Can you work these out from the model? Positions are in its coordinate system, mm. Face numbers are marked on the shaded views. Give positions to 0.01 mm unless a question says otherwise; leave off trailing zeros. Write each loop counter-clockwise with the first axis right and the second up, starting at its lowest first coordinate (ties: lowest second). Pieces come first, ordered by that corner, then holes. Notation, with made-up numbers: (83.5, -17) - (140.5, -17) arc R19 cw to (140.5, -8) - close; hole circle Ø7 at (-31.75, -27.75). An arc over 180 degrees is marked (long way). Return JSON: item names as keys, results as strings. Group by question number.
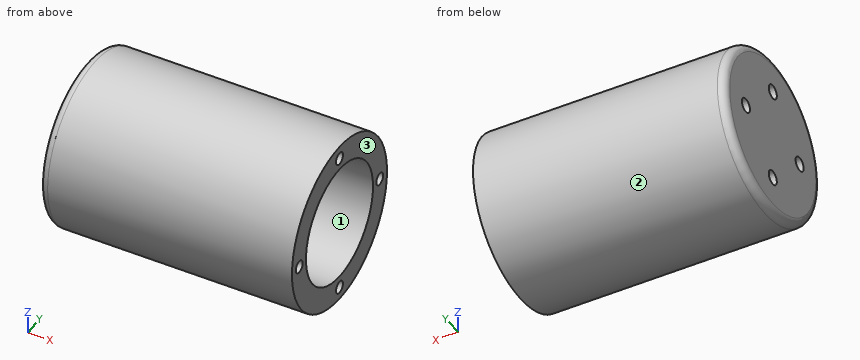
from build123d import *

# Parameters (mm, degrees)
SKETCH1_W          = 63.8
SKETCH1_H          = 21.25
SKETCH2_R          = 15
CUT_EXTRUDE1_DEPTH = 61.3
SKETCH3_R          = 1.55
CUT_EXTRUDE2_DEPTH = 3.8
CIRPATTERN1_COUNT  = 4
CUT_EXTRUDE3_REACH = 70.27
SKETCH4_R          = 1.8
CIRPATTERN2_COUNT  = 4
FILLET1_R          = 2


with BuildPart() as part:
    # Sketch1 → Revolve1 (revolve)
    with BuildSketch(Plane.XY, mode=Mode.PRIVATE) as revolve1_sk:
        with Locations((0, 10.625)):
            Rectangle(SKETCH1_W, SKETCH1_H)
    revolve(revolve1_sk.sketch.rotate(Axis((-31.9, 0, 0), (1, 0, 0)), 180), axis=Axis((-31.9, 0, 0), (1, 0, 0)))

    # Sketch2 → Cut-Extrude1 (cut)
    with BuildSketch(Plane(origin=(31.9, 0, 0), x_dir=(0, 0, -1), z_dir=(1, 0, 0))):
        with Locations(Location((0, 0, 0), (0, 0, 90))):
            Circle(SKETCH2_R)
    extrude(amount=-CUT_EXTRUDE1_DEPTH, mode=Mode.SUBTRACT)

    # Sketch3 → Cut-Extrude2 (cut)
    with BuildSketch(Plane(origin=(31.9, 0, 0), x_dir=(0, 0, -1), z_dir=(1, 0, 0))):
        with Locations(Location((0, 18, 0), (0, 0, 90))):
            Circle(SKETCH3_R)
    cut_extrude2 = extrude(amount=-CUT_EXTRUDE2_DEPTH, mode=Mode.SUBTRACT)

    # CirPattern1: Cut-Extrude2 ×4 about axis
    cirpattern1_axis = Axis((0, 0, 0), (1, 0, 0))
    for i in range(1, CIRPATTERN1_COUNT):
        add(cut_extrude2.rotate(cirpattern1_axis, i * 360 / CIRPATTERN1_COUNT), mode=Mode.SUBTRACT)

    # Sketch4 → Cut-Extrude3 (cut, up to next)
    with BuildSketch(Plane(origin=(-29.4, 0, 0), x_dir=(0, 0, -1), z_dir=(1, 0, 0)), mode=Mode.PRIVATE) as cut_extrude3_sk1:
        with Locations(Location((0, 12, 0), (0, 0, 90))):
            Circle(SKETCH4_R)
    cut_extrude3_tool1 = extrude(cut_extrude3_sk1.sketch, amount=-CUT_EXTRUDE3_REACH, mode=Mode.PRIVATE) & part.part
    cut_extrude3 = cut_extrude3_tool1.solids().sort_by_distance((-29.4, 12, 0))[0]
    add(cut_extrude3, mode=Mode.SUBTRACT)

    # CirPattern2: Cut-Extrude3 ×4 about axis
    cirpattern2_axis = Axis((0, 0, 0), (1, 0, 0))
    for i in range(1, CIRPATTERN2_COUNT):
        add(cut_extrude3.rotate(cirpattern2_axis, i * 360 / CIRPATTERN2_COUNT), mode=Mode.SUBTRACT)

    # Fillet1
    fillet1_edges = [part.edges().sort_by_distance(p)[0] for p in [
        (-31.9, 21.25, 0),
    ]]
    fillet(fillet1_edges, radius=FILLET1_R)


solid = part.part
1) Imagine slicing it at A-A, the plane y = 0. Write out the boundary of the cut face in (x, z).
2) We'd pull the mould along Y, two halves only. Please class the marked faces 1, 2 and 3: pulls with the +Y half, pulls with the -Y half, needs draft (parallel to the pull), parting line crosses it, or undercut.
3) Will these pins go through, and if not, where does the flat tip stop? pin 1 Ø0.9 at (y, z) = (-17.5, -0.5) entering from +X; pin 2 Ø8 at (x, z) = (-19, -6.5) entering from +Y; pin 3 Ø2 at (x, y) = (20.5, 2.5) entering from +Z; pin 4 Ø3 at (y, z) = (12, 0) entering from +X.
4) Imagine slicing it at B-B, the plane x = 18. Write out the boundary of the cut face in (y, z).
5) I need wall thicknesses on line 1 along Z through (x, y) = (-7, -0.5); line 2 along Z through (x, y) = (-17.5, 9); line 3 along Y through (x, z) = (13, -3). Which ranges of each line are inside material? Lowest first, please.
Resolved:
{
 "1": {"outline": "(-31.9, -19.25) arc R2 ccw to (-29.9, -21.25) - (31.9, -21.25) - (31.9, -19.55) - (28.1, -19.55) - (28.1, -16.45) - (31.9, -16.45) - (31.9, -15) - (-29.4, -15) - (-29.4, -13.8) - (-31.9, -13.8) - close; (-31.9, -10.2) - (-29.4, -10.2) - (-29.4, 10.2) - (-31.9, 10.2) - close; (-31.9, 13.8) - (-29.4, 13.8) - (-29.4, 15) - (31.9, 15) - (31.9, 16.45) - (28.1, 16.45) - (28.1, 19.55) - (31.9, 19.55) - (31.9, 21.25) - (-29.9, 21.25) arc R2 ccw to (-31.9, 19.25) - close"},
 "2": {"face 1": "undercut", "face 2": "parting line crosses it", "face 3": "needs draft"},
 "3": {"pin 1": "x = 28.1", "pin 2": "y = 21.1", "pin 3": "z = 21.2", "pin 4": "through"},
 "4": {"outline": "circle Ø42.5 at (0, 0); hole circle Ø30 at (0, 0)"},
 "5": {"line 1": "-21.24 to -14.99, 14.99 to 21.24", "line 2": "-19.25 to -12, 12 to 19.25", "line 3": "-21.04 to -14.7, 14.7 to 21.04"}
}
